Autodesk Inventor part; units mm, degrees
ref_plane "YZ Plane" through (0, 0, 0) normal (1, 0, 0) x (0, 1, 0)
ref_plane "XZ Plane" through (0, 0, 0) normal (0, 1, 0) x (-1, 0, 0)
ref_plane "XY Plane" through (0, 0, 0) normal (0, 0, 1) x (1, 0, 0)
sketch "草圖1" plane through (0, 0, 0) normal (0, 0, 1) x (1, 0, 0)
  arc A0 (0, 32.5) -> (0, -32.5) centre (0, 0) ccw
  arc A1 (0, 37.5) -> (0, -37.5) centre (0, 0) ccw
  arc A2 (0, 42.5) -> (0, -42.5) centre (0, 0) ccw
  line L0 (0, 0) -> (0, -59.8463)
  line L1 (0, -59.8463) -> (0, 72.1748)
  point P0 (0, -37.5)
  point P1 (0, -42.5)
  dimension "d16" = 32.5
  dimension "d17" = 37.5
  dimension "d18" = 42.5
extrude "擠出1" add sketch "草圖1" along normal blind 10 contours A0 L0 A1 L1
extrude "擠出2" add sketch "草圖1" along normal mid plane 20 contours A1 L0 A2 L1
sketch "草圖2" plane through (0, 0, 10) normal (0, 0, 1) x (1, 0, 0)
  line L0 (0, 32.5) -> (0, 42.5)
  line L1 (0, 42.5) -> (0, 52.5)
  arc A0 (0, 42.5) -> (0, -42.5) centre (0, 0) ccw
  line L2 (-16.411, 39.2037) -> (-16.411, 59.2037)
  line L3 (-16.411, 59.2037) -> (0, 59.2037)
  line L4 (0, 59.2037) -> (0, 42.5)
  dimension "d4" = 10
  dimension "d9" = 20
  dimension "d13" = 16.411
extrude "擠出3" add sketch "草圖2" against normal blind 10
sketch "草圖4" plane through (0, 0, 10) normal (0, 0, 1) x (1, 0, 0)
  line L0 (0, 59.2037) -> (0, 37.5)
  line L1 (-16.411, 59.2037) -> (-16.411, 39.2037)
  line L2 (-16.411, 59.2037) -> (-8.206, 59.2037)
  line L3 (-8.206, 59.2037) -> (-8.206, 56.2037)
  circle A0 centre (-8.206, 56.2037) radius 1.5
  point P0 (0, 0)
  dimension "d21" = 8.205
  dimension "d22" = 3
  dimension "d23" = 3
extrude "擠出4" cut sketch "草圖4" against normal blind 20
sketch "草圖5" plane through (0, 0, 10) normal (0, 0, 1) x (1, 0, 0)
  line L0 (-54.3449, 0) -> (9.0575, 0) construction
  line L1 (0, -52.5) -> (0, 52.5) construction
  line L2 (-45.2874, 15) -> (-41, 15)
  line L3 (-41, 15) -> (-41, -15)
  line L4 (-41, -15) -> (-45.2874, -15)
  line L5 (-45.2874, -15) -> (-45.2874, 15)
  point P0 (0, 0)
  dimension "d24" = 15
  dimension "d25" = 15
  dimension "d26" = 41
extrude "擠出5" cut sketch "草圖5" against normal blind 28
properties part number "ARMR"
Could you check a few things on this model? Use its own coordinates, in mm. A direction names the side the tool comes from. Give positions to 0.01 mm unless a question says otherwise; leave off trailing zeros. Loops run counter-clockwise (first coordinate to the right, second up) from the corner with the lowest first, then second, coordinate; pieces in that order, holes last. Notation, with made-up numbers: (70, -24) - (123, -24) arc R29 cw to (123, 3) - close; hole circle Ø10 at (3.25, 32.5). An arc over 180 degrees is marked (long way). Answer in a Markdown table with one row per item. Add a question column.
Q1. For pin 1 (5 mm diameter, centred on x = -28, y = 4, fed in from +Z); pin 2 (5 mm diameter, centred on x = -9.5, y = 48, fed in from -Z); pin 3 (1.5 mm diameter, centred on x = -13, z = 8, fed in from -Y); pin 4 (6 mm diameter, centred on y = -26.5, z = -4.5, fed in from -X), each with a flat end and sliding along its axis, tell me the tip position at first contact or that it passes through.
Q2. Which directions (+Z, -Z, +X, -X, +Y, -Y) give clear straight access to the entire face, cutting with the end or side of a thin tool? Please do faces 1 (the face through (-39, -3, -10)), 2 (the face through (-37.49, -0.82, -5.07)).
Q3. Please list where these lines run through material, in increasing order: L1, parallel to Y at x = -9.5, z = 6.25; L2, parallel to Z at x = -36, y = -3.5; L3, parallel to Y at x = -23, z = 4.75. Write a range as from..to.
Q4. If we section it at C-C (y = 0): List the corners of the cut face in (x, z) for me, plus the area to 3 significant figures.
Q5. If we section it at A-A (x = -21): List the corners of the cut face in (y, z) for me, plus the area to 3 significant figures.
Q6. If we section it at B-B (z = 6.5): List the corners of the cut face in (x, y) for me, plus the area to 3 significant figures.
Q7. We'd pull the mould along Y, two halves only. Please class faces 3 (the face through (-8, 59.204, 5)), 4 (the face through (-32.492, -0.715, 4.93)), 5 (the face through (-16.411, 49, 5)), 6 (the face through (-25.5, -34, -0.1)): +Y half, -Y half, draft (parallel to the pull), parting line (faces both ways), or undercut.
Q8. If we section it at D-D (x = -31.5): List the corners of the cut face in (y, z) for me.
The answers:
| question | item | result |
|---|---|---|
| 1 | pin 1 | passes through |
| 1 | pin 2 | stops at z = 0 |
| 1 | pin 3 | stops at y = -40.7 |
| 1 | pin 4 | stops at x = -35.41 |
| 2 | face 1 | -Z, +X, -X, +Y, -Y |
| 2 | face 2 | -Z, +X |
| 3 | L1 | y = -41.42..-31.08, 31.08..55.45, 56.96..59.2 |
| 3 | L2 | z = 0..10 |
| 3 | L3 | y = -35.74..-22.96, 22.96..35.74 |
| 4 | outline | (-41, -10) - (-37.5, -10) - (-37.5, 0) - (-32.5, 0) - (-32.5, 10) - (-41, 10) - close |
| 4 | area | 120 mm^2 |
| 5 | outline | (-36.95, -10) - (-31.07, -10) - (-31.07, 0) - (-24.8, 0) - (-24.8, 10) - (-36.95, 10) - close; (24.8, 0) - (31.07, 0) - (31.07, -10) - (36.95, -10) - (36.95, 10) - (24.8, 10) - close |
| 5 | area | 361 mm^2 |
| 6 | outline | (-41, -11.19) arc R42.5 ccw to (0, -42.5) - (0, -32.5) arc R32.5 cw to (0, 32.5) - (0, 59.2) - (-16.41, 59.2) - (-16.41, 39.2) arc R42.5 ccw to (-41, 11.19) - close; hole circle Ø3 at (-8.21, 56.2) |
| 6 | area | 1,440 mm^2 |
| 7 | face 3 | +Y half |
| 7 | face 4 | undercut |
| 7 | face 5 | draft |
| 7 | face 6 | -Y half |
| 8 | outline | (-28.53, -10) - (-20.35, -10) - (-20.35, 0) - (-8, 0) - (-8, 10) - (-28.53, 10) - close; (8, 0) - (20.35, 0) - (20.35, -10) - (28.53, -10) - (28.53, 10) - (8, 10) - close |
